Design review of the part built by this model. Coordinates are the model's own, in mm. A direction names the side the tool comes from. Coordinates: 2 decimals unless noted, no trailing zeros. Order: outer loops, then holes, each group sorted by start corner. A loop starts at its lowest first (then second) coordinate and runs counter-clockwise, first axis right, second up. Notation, with made-up numbers: (-37.75, 36) -> (-8.75, 36) arc R23 cw to (-8.75, 74) -> close; hole circle Ø4 at (29, 10). An arc over 180 degrees is marked (long way). Use a Markdown table: item, result. Add a question column.
Q1. Wall thickness on probe 1 along X at (y, z) = (0, 0.85); probe 2 along Y at (x, z) = (16.5, 0.6); probe 3 along Y at (x, z) = (0, 4.3): over which ranges is each line inside the solid? List them lowest first.
Q2. Add section B-B (x = 16.5). State the section outline as (y, z) points.
Q3. The part is to be moulded in two halves that separate along Y. For faces 3 (the face through (0, 0, 1.5)), 4 (the face through (29, 0, 1)), 5 (the face through (13, 0, 1.5)), say which applies: pulls with the +Y half, pulls with the -Y half, needs draft (parallel to the pull), parting line crosses it, or undercut.
Q4. Add section C-C (z = 4.75). State the section outline as (x, y) points.
Q5. Machinability: for faces 1 (the face through (13, 0, 0)), 2 (the face through (-1.5, -0.07, 3.96)), which of the approach directions +Z, -Z, +X, -X, +Y, -Y give a long, thin tool a straight path to every point of the face, cutting with its end or side? Answer none if there is none.
Q6. Add section D-D (x = 1). State the section outline as (y, z) points.
Q7. Add section A-A (y = 0). State the section outline as (x, z) points, then the cut area to 3 significant figures.
Q8. Insertion check: pin 1 (4 mm diameter, centred on x = 17.5, y = -0.5, fed in from +Z). The pin has a flat end and moves straight along its axis. Give the tip position at first contact, or say it passes through.
Autodesk Inventor part; units mm, degrees
ref_plane "YZ Plane" through (0, 0, 0) normal (1, 0, 0) x (0, 1, 0)
ref_plane "XZ Plane" through (0, 0, 0) normal (0, 1, 0) x (-1, 0, 0)
ref_plane "XY Plane" through (0, 0, 0) normal (0, 0, 1) x (1, 0, 0)
sketch "Эскиз1" plane through (0, 0, 0) normal (0, 0, 1) x (1, 0, 0)
  line L0 (0, 0) -> (25.5, 0) construction
  line L1 (0, -3.5) -> (25.5, -3.5)
  line L2 (25.5, 3.5) -> (0, 3.5)
  arc A0 (0, 3.5) -> (0, -3.5) centre (0, 0) ccw
  arc A1 (25.5, -3.5) -> (25.5, 3.5) centre (25.5, 0) ccw
  point P0 (12.75, 0)
  dimension "d0" = 25.5
  dimension "d1" = 7
extrude "Выдавливание1" add sketch "Эскиз1" along normal blind 1.5
sketch "Эскиз2" plane through (0, 0, 1.5) normal (0, 0, 1) x (1, 0, 0)
  circle A0 centre (0, 0) radius 2.5
  circle A1 centre (0, 0) radius 1.5
  dimension "d4" = 5
  dimension "d5" = 1
extrude "Выдавливание2" add sketch "Эскиз2" along normal blind 5
sketch "Эскиз6" plane through (0, 0, 0) normal (0, 0, 1) x (1, 0, 0)
  line L0 (-10, 0) -> (35.5, 0) construction
  arc A0 (25.5, -3.5) -> (25.5, 3.5) centre (25.5, 0) ccw construction
  circle A1 centre (26.5, 0) radius 0.5
  circle A2 centre (16.5, 0) radius 0.5
  point P0 (0, 0)
  point P1 (29, 0)
  point P2 (29, 0)
  dimension "d22" = 1
  dimension "d23" = 2.5
  dimension "d25" = 10
hole "Отверстие1" at (26.5, 0, 0) at (16.5, 0, 0) direction (0, 0, 1) diameter 1 end through all countersink diameter 1.5 countersink angle 90
properties part number "элемент-2"
Established:
| question | item | result |
|---|---|---|
| 1 | probe 1 | -3.5 to 16, 17 to 26, 27 to 29 |
| 1 | probe 2 | -3.5 to -0.5, 0.5 to 3.5 |
| 1 | probe 3 | -2.5 to -1.5, 1.5 to 2.5 |
| 2 | outline | (-3.5, 0) -> (-0.75, 0) -> (-0.5, 0.25) -> (-0.5, 1.5) -> (-3.5, 1.5) -> close; (0.5, 0.25) -> (0.75, 0) -> (3.5, 0) -> (3.5, 1.5) -> (0.5, 1.5) -> close |
| 3 | face 3 | undercut |
| 3 | face 4 | parting line crosses it |
| 3 | face 5 | needs draft |
| 4 | outline | circle Ø5 at (0, 0); hole circle Ø3 at (0, 0) |
| 5 | face 1 | -Z, +X, -X, +Y, -Y |
| 5 | face 2 | +Z |
| 6 | outline | (-3.5, 0) -> (3.5, 0) -> (3.5, 1.5) -> (2.29, 1.5) -> (2.29, 6.5) -> (1.12, 6.5) -> (1.12, 1.5) -> (-1.12, 1.5) -> (-1.12, 6.5) -> (-2.29, 6.5) -> (-2.29, 1.5) -> (-3.5, 1.5) -> close |
| 7 | outline | (-3.5, 0) -> (15.75, 0) -> (16, 0.25) -> (16, 1.5) -> (2.5, 1.5) -> (2.5, 6.5) -> (1.5, 6.5) -> (1.5, 1.5) -> (-1.5, 1.5) -> (-1.5, 6.5) -> (-2.5, 6.5) -> (-2.5, 1.5) -> (-3.5, 1.5) -> close; (17, 0.25) -> (17.25, 0) -> (25.75, 0) -> (26, 0.25) -> (26, 1.5) -> (17, 1.5) -> close; (27, 0.25) -> (27.25, 0) -> (29, 0) -> (29, 1.5) -> (27, 1.5) -> close |
| 7 | area | 55.6 mm^2 |
| 8 | pin 1 | z = 1.5 |
